Geometry: final body of the model. Coordinates: model frame, mm. A direction names the side the tool comes from. Give positions to 0.01 mm unless a question says otherwise; leave off trailing zeros. Write each loop counter-clockwise with the first axis right and the second up, starting at its lowest first coordinate (ties: lowest second). Pieces come first, ordered by that corner, then holes.
from build123d import *

# Parameters (mm, degrees)
F2_R     = 25.625
F3_DEPTH = 2
F5_DEPTH = 2
F6_R     = 4.99999
F7_R     = 3


# Not quite as in the source:
# - a fillet or chamfer is up to 0.001 mm smaller than in the source, because OpenCascade refuses the exact size


with BuildPart() as f1:
    # F0 (on Top) → F1 (revolve)
    with BuildSketch(Plane.XY):
        Polygon((-18.3333333333, 18.75), (-18.3333333333, 13.75), (0, 13.75), (11.907849302, 20.625), (25.657849302, 20.625), (25.657849302, 25.625), (10.5681033399, 25.625), (-1.3397459622, 18.75), align=None)
    revolve(axis=Axis((-8.7595172226, 0, 0), (1, 0, 0)))

    # F2 (on face) → F3 (join)
    with BuildSketch(Plane.YZ.offset(25.657849302)):
        Circle(F2_R)
    extrude(amount=F3_DEPTH)

    # F4 (on face) → F5 (cut, through all)
    with BuildSketch(Plane.YZ.offset(27.657849302)):
        with BuildLine():
            ThreePointArc((20.625, 0), (20.0867260274, 4.6812458278), (18.5, 9.1181481124))
            Line((18.5, 9.1181481124), (18.5, -9.1181481124))
            ThreePointArc((18.5, -9.1181481124), (20.0867260274, -4.6812458278), (20.625, 0))
        make_face()
        with BuildLine():
            ThreePointArc((17.5, 10.9151557479), (16.1096351924, 12.8790635905), (14.5, 14.6676727875))
            Line((14.5, 14.6676727875), (14.5, -14.6676727875))
            ThreePointArc((14.5, -14.6676727875), (16.1096351924, -12.8790635905), (17.5, -10.9151557479))
            Line((17.5, -10.9151557479), (17.5, 10.9151557479))
        make_face()
        with BuildLine():
            ThreePointArc((13.5, 15.5929671647), (12.0484676296, 16.7399239179), (10.5, 17.7522005678))
            Line((10.5, 17.7522005678), (10.5, -17.7522005678))
            ThreePointArc((10.5, -17.7522005678), (12.0484676296, -16.7399239179), (13.5, -15.5929671647))
            Line((13.5, -15.5929671647), (13.5, 15.5929671647))
        make_face()
        with BuildLine():
            ThreePointArc((9.5, 18.3068463969), (8.0250486473, 18.9997162929), (6.5, 19.573978262))
            Line((6.5, 19.573978262), (6.5, -19.573978262))
            ThreePointArc((6.5, -19.573978262), (8.0250486473, -18.9997162929), (9.5, -18.3068463969))
            Line((9.5, -18.3068463969), (9.5, 18.3068463969))
        make_face()
        with BuildLine():
            ThreePointArc((5.5, 19.8781444054), (4.0110398588, 20.2312180615), (2.5, 20.4729241927))
            Line((2.5, 20.4729241927), (2.5, -20.4729241927))
            ThreePointArc((2.5, -20.4729241927), (4.0110398588, -20.2312180615), (5.5, -19.8781444054))
            Line((5.5, -19.8781444054), (5.5, 19.8781444054))
        make_face()
        with BuildLine():
            ThreePointArc((1.5, 20.5703822279), (0.7504970188, 20.6113410341), (0, 20.625))
            ThreePointArc((0, 20.625), (-0.7504970188, 20.6113410341), (-1.5, 20.5703822279))
            Line((-1.5, 20.5703822279), (-1.5, -20.5703822279))
            ThreePointArc((-1.5, -20.5703822279), (-0.7504970188, -20.6113410341), (0, -20.625))
            ThreePointArc((0, -20.625), (0.7504970188, -20.6113410341), (1.5, -20.5703822279))
            Line((1.5, -20.5703822279), (1.5, 20.5703822279))
        make_face()
        with BuildLine():
            Line((-2.5, -20.4729241927), (-2.5, 20.4729241927))
            ThreePointArc((-2.5, 20.4729241927), (-4.0110398588, 20.2312180615), (-5.5, 19.8781444054))
            Line((-5.5, 19.8781444054), (-5.5, -19.8781444054))
            ThreePointArc((-5.5, -19.8781444054), (-4.0110398588, -20.2312180615), (-2.5, -20.4729241927))
        make_face()
        with BuildLine():
            Line((-6.5, -19.573978262), (-6.5, 19.573978262))
            ThreePointArc((-6.5, 19.573978262), (-8.0250486473, 18.9997162929), (-9.5, 18.3068463969))
            Line((-9.5, 18.3068463969), (-9.5, -18.3068463969))
            ThreePointArc((-9.5, -18.3068463969), (-8.0250486473, -18.9997162929), (-6.5, -19.573978262))
        make_face()
        with BuildLine():
            Line((-10.5, -17.7522005678), (-10.5, 17.7522005678))
            ThreePointArc((-10.5, 17.7522005678), (-12.0484676296, 16.7399239179), (-13.5, 15.5929671647))
            Line((-13.5, 15.5929671647), (-13.5, -15.5929671647))
            ThreePointArc((-13.5, -15.5929671647), (-12.0484676296, -16.7399239179), (-10.5, -17.7522005678))
        make_face()
        with BuildLine():
            Line((-14.5, -14.6676727875), (-14.5, 14.6676727875))
            ThreePointArc((-14.5, 14.6676727875), (-16.1096351924, 12.8790635905), (-17.5, 10.9151557479))
            Line((-17.5, 10.9151557479), (-17.5, -10.9151557479))
            ThreePointArc((-17.5, -10.9151557479), (-16.1096351924, -12.8790635905), (-14.5, -14.6676727875))
        make_face()
        with BuildLine():
            Line((-18.5, -9.1181481124), (-18.5, 9.1181481124))
            ThreePointArc((-18.5, 9.1181481124), (-20.625, 0), (-18.5, -9.1181481124))
        make_face()
    extrude(amount=-F5_DEPTH, mode=Mode.SUBTRACT)

    # F6 (radius 5 in the source; OpenCascade refuses exactly that, so slightly less here)
    f6_edges = [f1.edges().sort_by_distance(p)[0] for p in [
        (-18.333333, -18.75, 0),
        (-1.339746, -18.75, 0),
        (10.568103, -25.625, 0),
    ]]
    fillet(f6_edges, radius=F6_R)

    # F7
    f7_edges = [f1.edges().sort_by_distance(p)[0] for p in [
        (11.907849, -20.625, 0),
        (0, -13.75, 0),
    ]]
    fillet(f7_edges, radius=F7_R)


solid = f1.part
Q1. Pull-direction query (Y, two-part tool) for faces 1 (the flat face through (27, 1.5, 0)), 2 (the conical face through (0.286, 18.779, 5.914)), 3 (the flat face through (27, -6.5, 0)), 4 (the flat face through (27.658, -6, 0)); classes: released by +Y, released by -Y, zero draft, split by the parting line, or undercut.
Filled sheet:
face 1: undercut
face 2: split by the parting line
face 3: undercut
face 4: zero draft
Q2. Ray query, line 1 along Y through (x, z) = (16.5, -0.5); line 2 along Y through (x, z) = (-4, 0); line 3 along Z through (x, y) = (16, 0) (3 decimals). Return the intervals inside material, ascending.
Filled sheet:
line 1: y = -25.62 to -20.62, 20.62 to 25.62
line 2: y = -18.75 to -13.75, 13.75 to 18.75
line 3: z = -25.625 to -20.625, 20.625 to 25.625
Q3. Access query for faces 5 (the cylindrical face through (-8.081, 17.884, 5.632)), 6 (the cylindrical face through (19.673, 23.671, -9.815)), 7 (the flat face through (27, 14.5, 0)). Directions: +Z, -Z, +X, -X, +Y, -Y. A direction counts if a zero-diameter tool reaches every point of the face in a straight line with its end or side. Return the directions, or none.
Filled sheet:
face 5: -X
face 6: +X, -X
face 7: +X
Q4. Pin query (flat end, axial travel): P1, Ø2, axis at x = 0, y = -3, coming from the -Z side; P2, Ø0.5, axis at y = 6, z = -7, coming from the -X side; P3, Ø8, axis at x = -6, z = -20.5, coming from the -Y side; P4, Ø2, axis at x = 26.5, z = -0.5, coming from the +Y side (3 decimals). Return the tip coordinate at first contact, or that it passes through.
Filled sheet:
P1: stops at z = -19.89
P2: stops at x = 25.66
P3: stops at y = -8.91
P4: stops at y = 25.625
Q5. Section B-B on x = -7. Output: boundary loops of the cut face in (y, z), plus the area to 3 significant figures.
Filled sheet:
outline: circle Ø37.5 at (0, 0); hole circle Ø27.5 at (0, 0)
area: 511 mm2
Q6. Section A-A on x = 14.5. Output: boundary loops of the cut face in (y, z) (3 decimals), plus the area to 3 significant figures.
Filled sheet:
outline: circle Ø51.25 at (0, 0); hole circle Ø41.25 at (0, 0)
area: 726 mm2
